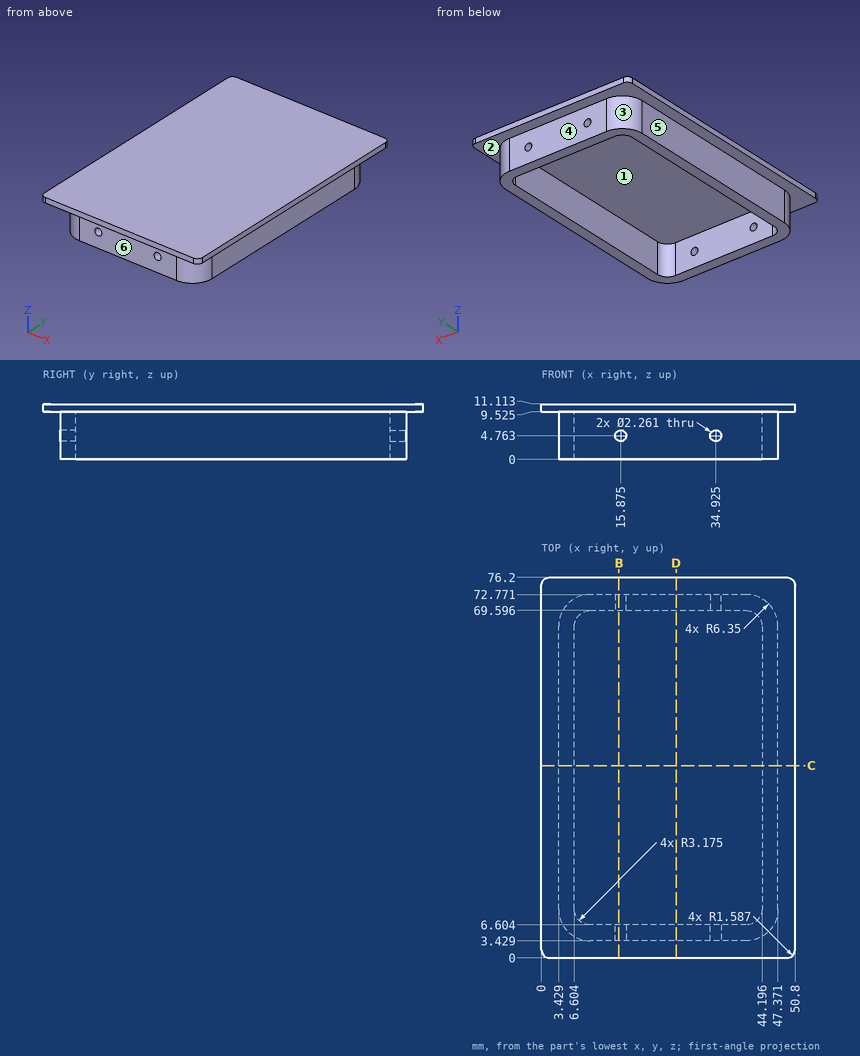
Part print with two shaded views. Sizes in mm from the minimum x, y, z corner. A direction names the side the tool comes from. Coordinates: 2 decimals unless noted, no trailing zeros. Order: outer loops, then holes, each group sorted by start corner. A loop starts at its lowest first (then second) coordinate and runs counter-clockwise, first axis right, second up. Notation, with made-up numbers: M -27.5,38.25 L 13.5,38.25 A19 ccw 13.5,69.25 Z; hole C 9.25,-11.75 d10. An arc over 180 degrees is marked long. Use a Markdown table: item, result.
(1) Cut at D-D on x = 27. Write the cut outline in (y, z) (1 decimal).
A:
| item | result |
|---|---|
| outline | M 0,9.5 L 3.4,9.5 L 3.4,0 L 6.6,0 L 6.6,9.5 L 69.6,9.5 L 69.6,0 L 72.8,0 L 72.8,9.5 L 76.2,9.5 L 76.2,11.1 L 0,11.1 Z |
(2) Flat gauge pins, fed straight in: pin 1 (5 mm diameter, centred on x = 27, z = 4.5, fed in from -Y); pin 2 (2 mm diameter, centred on x = 18.5, y = 47.5, fed in from -Z) (1 decimal); pin 3 (3 mm diameter, centred on x = 15.87, z = 4.76, fed in from +Y). Where does each tip first touch, or does it go through?
A:
| item | result |
|---|---|
| pin 1 | stops at y = 3.43 |
| pin 2 | stops at z = 9.5 |
| pin 3 | stops at y = 72.77 |
(3) Cut at B-B on x = 15.5. Write the cut outline in (y, z) (1 decimal), then the cut area to 3 significant figures.
A:
| item | result |
|---|---|
| outline | M 0,9.5 L 3.4,9.5 L 3.4,5.8 L 6.6,5.8 L 6.6,9.5 L 69.6,9.5 L 69.6,5.8 L 72.8,5.8 L 72.8,9.5 L 76.2,9.5 L 76.2,11.1 L 0,11.1 Z; M 3.4,0 L 6.6,0 L 6.6,3.7 L 3.4,3.7 Z; M 69.6,0 L 72.8,0 L 72.8,3.7 L 69.6,3.7 Z |
| area | 168 mm^2 |
(4) Probe L1, parallel to X at y = 32, z = 9 (1 decimal); L2, parallel to Y at x = 26.5, z = 2.75 (1 decimal); L3, parallel to Z at x = 3, y = 44.5 (1 decimal). List the from-to ranges inside material, lowest first.
A:
| item | result |
|---|---|
| L1 | x = 3.4 to 6.6, 44.2 to 47.4 |
| L2 | y = 3.4 to 6.6, 69.6 to 72.8 |
| L3 | z = 9.5 to 11.1 |
(5) Pull direction Y, two halves, no side cores. Call the marked faces 1, 2 and 3: released by +Y, released by -Y, zero draft, split by the parting line, or undercut.
A:
| item | result |
|---|---|
| face 1 | undercut |
| face 2 | zero draft |
| face 3 | released by +Y |
(6) Tool access for the marked faces 4, 5 and 6: list every direction of +Z, -Z, +X, -X, +Y, -Y with a clear straight run to the whole face (end or side of a thin tool).
A:
| item | result |
|---|---|
| face 4 | -Z, +X, -X, +Y |
| face 5 | -Z, -X, +Y, -Y |
| face 6 | -Z, +X, -X, -Y |
(7) Cut at C-C on y = 38.5. Write the cut outline in (x, z) (1 decimal), then the cut area to 3 significant figures.
A:
| item | result |
|---|---|
| outline | M 0,9.5 L 3.4,9.5 L 3.4,0 L 6.6,0 L 6.6,9.5 L 44.2,9.5 L 44.2,0 L 47.4,0 L 47.4,9.5 L 50.8,9.5 L 50.8,11.1 L 0,11.1 Z |
| area | 141 mm^2 |
